Autodesk Inventor part; units mm, degrees
ref_plane "YZ Plane" through (0, 0, 0) normal (1, 0, 0) x (0, 1, 0)
ref_plane "XZ Plane" through (0, 0, 0) normal (0, 1, 0) x (-1, 0, 0)
ref_plane "XY Plane" through (0, 0, 0) normal (0, 0, 1) x (1, 0, 0)
sketch "Sketch1" plane through (0, 0, 0) normal (0, 0, 1) x (1, 0, 0)
  line L0 (-20, -32.6) -> (20, -32.6)
  line L1 (20, -32.6) -> (20, 32.6)
  line L2 (20, 32.6) -> (-20, 32.6)
  line L3 (-20, 32.6) -> (-20, -32.6)
  line L4 (-20, -32.6) -> (20, 32.6) construction
  line L5 (20, -32.6) -> (-20, 32.6) construction
  point P0 (0, 0)
  dimension "d0" = 40
  dimension "d1" = 65.2
extrude "Extrusion1" add sketch "Sketch1" along normal blind 10
sketch "Sketch2" plane through (-20, 32.6, 0) normal (0, 1, 0) x (1, 0, 0)
  line L0 (40, -10) -> (40, -5)
  line L1 (40, 0) -> (40, -10)
  line L2 (40, -5) -> (35, -5)
  circle A0 centre (35, -5) radius 2
  line L3 (20, 0) -> (20, -10)
  circle A1 centre (5, -5) radius 2
  dimension "d4" = 5
  dimension "d5" = 5
  dimension "d6" = 4
extrude "Extrusion2" cut sketch "Sketch2" against normal blind 25
mirror "Mirror1" about plane through (0, 0, 0) normal (0, 1, 0) of "Extrusion2"
thread "Thread1"
thread "Thread2"
thread "Thread3"
thread "Thread4"
sketch "Sketch3" plane through (20, -32.6, 0) normal (1, 0, 0) x (0, 0, -1)
  line L0 (0, 32.6) -> (-5, 32.6)
  circle A0 centre (-5, 32.6) radius 2
  dimension "d17" = 5
  dimension "d18" = 4
extrude "Extrusion3" cut sketch "Sketch3" against normal blind 10
mirror "Mirror2" about plane through (0, 0, 0) normal (1, 0, 0) of "Extrusion3"
sketch "Sketch4" plane through (0, 0, 10) normal (0, 0, 1) x (1, 0, 0)
  point P0 (0, 0)
sketch "Sketch5" plane through (0, 0, 10) normal (0, 0, 1) x (1, 0, 0)
  line L0 (-20, -32.6) -> (20, -32.6)
  line L1 (0, -32.6) -> (0, 1.6)
  circle A0 centre (0, 1.6) radius 7.5
  line L2 (0, 1.6) -> (13, 1.6)
  point P0 (0, 0)
  dimension "d21" = 34.2
  dimension "d22" = 15
thread "Thread5"
thread "Thread6"
extrude "Extrusion6" cut sketch "Sketch5" against normal blind 10
sketch "Sketch6" plane through (0, 0, 10) normal (0, 0, 1) x (1, 0, 0)
  circle A0 centre (13, 6.6) radius 3.75
sketch "Boceto7" plane through (0, 0, 0) normal (0, 0, -1) x (-1, 0, 0)
  circle A0 centre (0, 1.6) radius 3.9163
  circle A1 centre (0, 1.6) radius 7.5
  line L0 (0, 1.6) -> (9.5, 1.6)
  line L1 (9.5, 1.6) -> (9.5, 7.6)
  circle A2 centre (9.5, 7.6) radius 2.5
  point P0 (0, 0)
  dimension "d38" = 9.5
  dimension "d39" = 6
  dimension "d40" = 5
extrude "Extrusión7" cut sketch "Boceto7" against normal blind 10 contours A2
sketch "Boceto8" plane through (0, 0, 10) normal (0, 0, 1) x (1, 0, 0)
  circle A0 centre (-9.5, 7.6) radius 2.5
sketch "Boceto9" plane through (0, 0, 0) normal (0, 0, -1) x (-1, 0, 0)
  circle A0 centre (9.5, 7.6) radius 2.5
sketch "Boceto10" plane through (0, 0, 10) normal (0, 0, 1) x (1, 0, 0)
  circle A0 centre (-9.5, 7.6) radius 2.5
sketch "Boceto11" plane through (0, 0, 0) normal (0, 0, -1) x (-1, 0, 0)
  circle A0 centre (9.5, 7.6) radius 2.5
properties part number "Rb PEEK - Corto con ventana"
Build history of the part. All positions in model axes, mm. A direction names the side the tool comes from. Give positions to 0.01 mm unless a question says otherwise; leave off trailing zeros. Loops run counter-clockwise (first coordinate to the right, second up) from the corner with the lowest first, then second, coordinate; pieces in that order, holes last. Notation, with made-up numbers: (0.5, 25) - (46.5, 25) arc R33 ccw to (46.5, 60) - close; hole circle Ø3 at (44, 85.25). An arc over 180 degrees is marked (long way). Use a Markdown table: item, result.
(1) Band-saw the part on B-B (z = 5). Give the number of separate pieces and of enclosed holes in the cut face, and give its area (3 significant figures).
Taken from the geometry:
| item | result |
|---|---|
| separate pieces | 1 |
| enclosed holes | 2 |
| area | 1,930 mm2 |
(2) Which spindle directions (+Z, -Z, +X, -X, +Y, -Y) get a long thin tool onto all of the face, cutting with end or side? Do faces 4 (the face through (15, 7.6, 5)), 5 (the face through (-20, 0.5, 2.7)), 6 (the face through (-15, -20, 7)), 7 (the face through (10, 0, 5)), 8 (the face through (-10, 0, 5)). Say none if no direction does.
Taken from the geometry:
| item | result |
|---|---|
| face 4 | +Y |
| face 5 | +Z, -Z, -X, +Y, -Y |
| face 6 | -Y |
| face 7 | +X |
| face 8 | -X |
(3) Band-saw the part on C-C (y = 0). Give the cut face in (x, z).
Taken from the geometry:
| item | result |
|---|---|
| outline | (-20, 0) - (-7.33, 0) - (-7.33, 10) - (-20, 10) - (-20, 7) - (-10, 7) - (-10, 3) - (-20, 3) - close; (7.33, 0) - (20, 0) - (20, 3) - (10, 3) - (10, 7) - (20, 7) - (20, 10) - (7.33, 10) - close |
(4) Wall check: line 1 along X through (y, z) = (22, 4.75); line 2 along Y through (x, z) = (15.25, 5); line 3 along X through (y, z) = (-25.5, 5.5). Give the ranges that are in metal, low to high.
Taken from the geometry:
| item | result |
|---|---|
| line 1 | -20 to -16.98, -13.02 to 13.02, 16.98 to 20 |
| line 2 | -7.6 to -2, 2 to 7.6 |
| line 3 | -20 to -16.94, -13.06 to 13.06, 16.94 to 20 |
(5) Drop flat-ended pins along their axis: pin 1 Ø3 at (x, z) = (15, 5) entering from -Y; pin 2 Ø2.5 at (y, z) = (0, 5) entering from -X; pin 3 Ø3.5 at (x, z) = (15, 5) entering from +Y. Give the stop position or say it passes through.
Taken from the geometry:
| item | result |
|---|---|
| pin 1 | y = -7.6 |
| pin 2 | x = -10 |
| pin 3 | y = 7.6 |
(6) Band-saw the part on D-D (y = -22.5). Give the cut face in (x, z), and give its area (3 significant figures).
Taken from the geometry:
| item | result |
|---|---|
| outline | (-20, 0) - (20, 0) - (20, 10) - (-20, 10) - close; hole circle Ø4 at (-15, 5); hole circle Ø4 at (15, 5) |
| area | 375 mm2 |
(7) Pull direction Y, two halves, no side cores. Call faces 1 (the face through (15.1, -1.2, 6.6)), 2 (the face through (-15, 7.6, 5)), 3 (the face through (20, -0.5, 2.7)): +Y half, -Y half, draft (parallel to the pull), parting line (faces both ways), or undercut.
Taken from the geometry:
| item | result |
|---|---|
| face 1 | undercut |
| face 2 | +Y half |
| face 3 | draft |
(8) Band-saw the part on A-A (x = -15). Give the cut face in (y, z).
Taken from the geometry:
| item | result |
|---|---|
| outline | (-32.6, 0) - (32.6, 0) - (32.6, 3) - (7.6, 3) - (7.6, 7) - (32.6, 7) - (32.6, 10) - (-32.6, 10) - (-32.6, 7) - (-7.6, 7) - (-7.6, 3) - (-32.6, 3) - close; hole circle Ø4 at (0, 5) |
